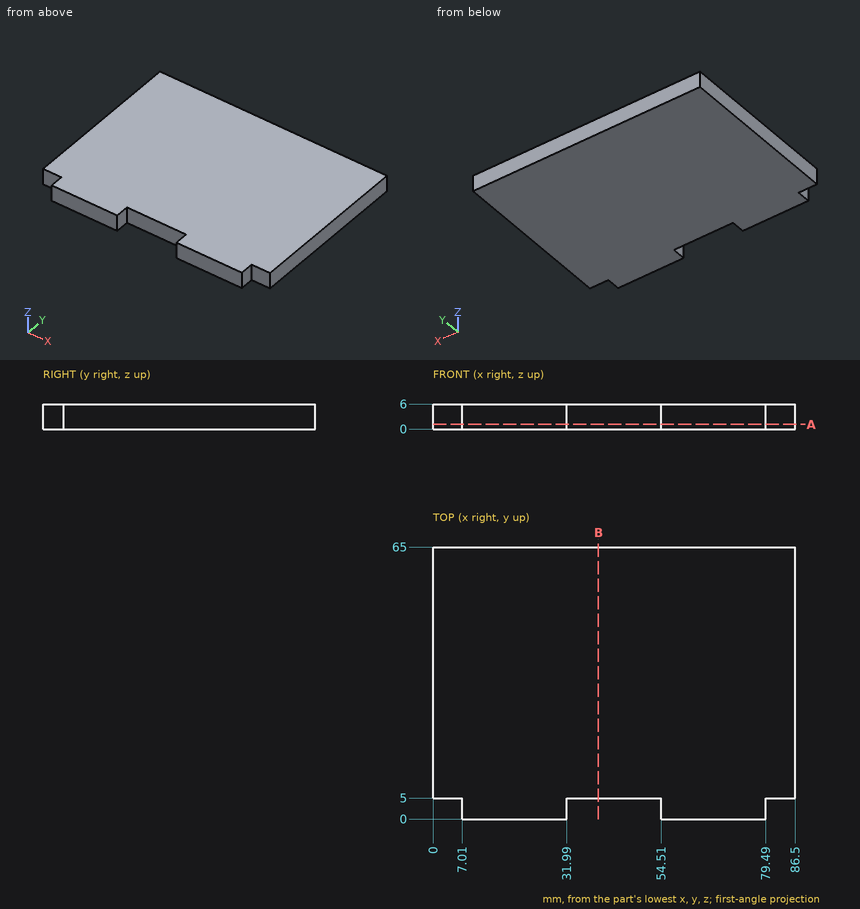
Design review of the part shown in the three views and the two pictorial views. Dimensions are in mm from the part's minimum x, y and z. Round coordinates to 2 decimals unless told otherwise and drop trailing zeros. Write each loop counter-clockwise with the first axis right and the second up, starting at its lowest first coordinate (ties: lowest second). Pieces come first, ordered by that corner, then holes. Notation, with made-up numbers: M 82.5,58 L 95.5,58 A21 ccw 95.5,79 Z; hole C 52,37.5 d5. An arc over 180 degrees is marked long. Use a Markdown table: item, result. Add a question column.
Q1. To check wall thickness, follow line 1 (Y direction, x = 48.5, z = 1.85). State the ranges of the line that lie inside material, in increasing order.
Q2. We need section B-B, the plane x = 39.5. State the section outline as (y, z) points.
Q3. Insertion check: pin 1 (2.5 mm diameter, centred on y = 1.5, z = 1.5, fed in from -X); pin 2 (3 mm diameter, centred on x = 84, z = 3.5, fed in from -Y); pin 3 (1.5 mm diameter, centred on y = 2.5, z = 3, fed in from +X). Each pin has a flat end and moves straight along its axis. Give the tip position at first contact, or say it passes through.
Q4. We need section A-A, the plane z = 1.15. State the section outline as (x, y) points.
Findings below:
| question | item | result |
|---|---|---|
| 1 | line 1 | y = 5 to 65 |
| 2 | outline | M 5,0 L 65,0 L 65,6 L 5,6 Z |
| 3 | pin 1 | stops at x = 7.01 |
| 3 | pin 2 | stops at y = 5 |
| 3 | pin 3 | stops at x = 79.49 |
| 4 | outline | M 0,5 L 7.01,5 L 7.01,0 L 31.99,0 L 31.99,5 L 54.51,5 L 54.51,0 L 79.49,0 L 79.49,5 L 86.5,5 L 86.5,65 L 0,65 Z |
